Design review of the part built by this model. Coordinates are the model's own, in mm. A direction names the side the tool comes from. Round coordinates to 2 decimals unless told otherwise and drop trailing zeros. Order: outer loops, then holes, each group sorted by start corner. A loop starts at its lowest first (then second) coordinate and runs counter-clockwise, first axis right, second up. Notation, with made-up numbers: (-25, 83.25) - (4, 83.25) arc R29 ccw to (4, 115.25) - close; hole circle Ø2 at (31.5, 32). An arc over 180 degrees is marked (long way). Answer as a JSON object with one key per item and string values. Group by question number.
from build123d import *

# Parameters (mm, degrees)
F1_DEPTH = 15
F3_DEPTH = 25


with BuildPart() as f1:
    # F0 (on Top) → F1 (new body)
    with BuildSketch(Plane.XY):
        with BuildLine():
            Line((0, 30), (0, 0))
            Line((0, 0), (18, 0))
            Line((18, 0), (18, 30))
            ThreePointArc((18, 30), (16.535534, 33.535534), (13, 35))
            Line((13, 35), (5, 35))
            ThreePointArc((5, 35), (1.464466, 33.535534), (0, 30))
        make_face()
    extrude(amount=F1_DEPTH)

    # F2 (on face) → F3 (join)
    with BuildSketch(Plane.XZ):
        with BuildLine():
            ThreePointArc((16.405338, 8.951662), (15.526659, 11.072982), (13.405338, 11.951662))
            Line((13.405338, 11.951662), (4.594662, 11.951662))
            ThreePointArc((4.594662, 11.951662), (2.473341, 11.072982), (1.594662, 8.951662))
            Line((1.594662, 8.951662), (1.594662, 6.048338))
            ThreePointArc((1.594662, 6.048338), (2.473341, 3.927018), (4.594662, 3.048338))
            Line((4.594662, 3.048338), (13.405338, 3.048338))
            ThreePointArc((13.405338, 3.048338), (15.526659, 3.927018), (16.405338, 6.048338))
            Line((16.405338, 6.048338), (16.405338, 8.951662))
        make_face()
    extrude(amount=F3_DEPTH)


solid = f1.part
1. Tool access review of faces 1 (the cylindrical face through (15.5, -12.3, 3.9)), 2 (the flat face through (9, -12, 3.048)), 3 (the flat face through (1.595, -12, 8)), 4 (the flat face through (16.405, -12, 7)): name each direction out of +Z, -Z, +X, -X, +Y, -Y from which nothing blocks a thin tool from reaching the whole face with its end or side.
2. Take a section at A-A, the plane z = 8.25. Give the boundary of the cut face in (x, y), then the cut area to 3 significant figures.
3. Take a section at C-C, the plane x = 11.25. Give the boundary of the cut face in (y, z).
4. Take a section at B-B, the plane y = -13. Give the boundary of the cut face in (x, z).
5. Take a section at D-D, the plane z = 13. Give the boundary of the cut face in (x, y), then the cut area to 3 significant figures.
6. To check wall thickness, follow line 1 (X direction, y = -9.5, z = 7.75); line 2 (Z direction, x = 10, y = -3.5); line 3 (Y direction, x = 13, z = 1). State the ranges of each line that lie inside material, in increasing order. Write a range as from..to.
7. Clearance check with flat-ended pins moving along their axes: P1, Ø9.5, axis at x = 10, y = -14.5, coming from the +Z side; P2, Ø1.5, axis at x = 16, y = -14.5, coming from the -Z side; P3, Ø2.5, axis at x = 9, y = -12.5, coming from the -Z side. State where each tip first meets the part, or that it passes through.
Response values:
{
 "1": {"face 1": "-Z, +X, -Y", "face 2": "-Z, +X, -X, -Y", "face 3": "+Z, -Z, -X, -Y", "face 4": "+Z, -Z, +X, -Y"},
 "2": {"outline": "(0, 0) - (1.59, 0) - (1.59, -25) - (16.41, -25) - (16.41, 0) - (18, 0) - (18, 30) arc R5 ccw to (13, 35) - (5, 35) arc R5 ccw to (0, 30) - close", "area": "990 mm2"},
 "3": {"outline": "(-25, 3.05) - (0, 3.05) - (0, 0) - (35, 0) - (35, 15) - (0, 15) - (0, 11.95) - (-25, 11.95) - close"},
 "4": {"outline": "(1.59, 6.05) arc R3 ccw to (4.59, 3.05) - (13.41, 3.05) arc R3 ccw to (16.41, 6.05) - (16.41, 8.95) arc R3 ccw to (13.41, 11.95) - (4.59, 11.95) arc R3 ccw to (1.59, 8.95) - close"},
 "5": {"outline": "(0, 0) - (18, 0) - (18, 30) arc R5 ccw to (13, 35) - (5, 35) arc R5 ccw to (0, 30) - close", "area": "619 mm2"},
 "6": {"line 1": "1.59..16.41", "line 2": "3.05..11.95", "line 3": "0..35"},
 "7": {"P1": "z = 11.95", "P2": "z = 3.68", "P3": "z = 3.05"}
}
